For this review, take the finished solid that the model builds, in its own axes (mm). A direction names the side the tool comes from. Give positions to 0.01 mm unless a question says otherwise; leave off trailing zeros. Loops run counter-clockwise (first coordinate to the right, second up) from the corner with the lowest first, then second, coordinate; pieces in that order, holes last. Notation, with made-up numbers: (61, 27) - (108, 27) arc R26 cw to (108, 51) - close; hole circle Ø11 at (30, -19.75). An arc over 180 degrees is marked (long way). Answer as CSV lines item,"result".
from build123d import *

# Parameters (mm, degrees)
BOSS_EXTRUDE1_DEPTH = 19
BOSS_EXTRUDE2_DEPTH = 9
SKETCH2_R           = 4.5
BOSS_EXTRUDE3_DEPTH = 60
CUT_EXTRUDE1_START  = -18
CUT_EXTRUDE1_DEPTH  = 18
CUT_EXTRUDE2_START  = -68
SKETCH4_R           = 4.511504631
SKETCH4_R_2         = 4.5
CUT_EXTRUDE2_DEPTH  = 68
CUT_EXTRUDE3_DEPTH  = 34
FILLET1_R           = 10
FILLET2_R           = 3


with BuildPart() as part:
    # Sketch1 → Boss-Extrude1 (new, symmetric)
    with BuildSketch(Plane.XY):
        with BuildLine():
            Line((-36, 0), (-27, 0))
            ThreePointArc((-27, 0), (0, -27), (27, 0))
            Line((27, 0), (36, 0))
            ThreePointArc((36, 0), (0, -36), (-36, 0))
        make_face()
    extrude(amount=BOSS_EXTRUDE1_DEPTH, both=True)

    # Sketch1<3> → Boss-Extrude2 (add, symmetric)
    with BuildSketch(Plane.XY):
        with BuildLine():
            ThreePointArc((-36, 0), (0, -36), (36, 0))
            Line((36, 0), (36, -60))
            Line((36, -60), (-36, -60))
            Line((-36, -60), (-36, 0))
        make_face()
    extrude(amount=BOSS_EXTRUDE2_DEPTH, both=True)

    # Sketch2 → Boss-Extrude3 (add)
    with BuildSketch(Plane.XZ.offset(60)):
        with BuildLine():
            Line((-38, 9), (38, 9))
            ThreePointArc((38, 9), (47, 0), (38, -9))
            Line((38, -9), (-38, -9))
            ThreePointArc((-38, -9), (-47, 0), (-38, 9))
        make_face()
        with Locations((-38, 0)):
            Circle(SKETCH2_R, mode=Mode.SUBTRACT)
        with Locations((38, 0)):
            Circle(SKETCH2_R, mode=Mode.SUBTRACT)
    extrude(amount=-BOSS_EXTRUDE3_DEPTH)

    # Sketch3 → Cut-Extrude1 (cut)
    with BuildSketch(Plane(origin=(0, 0, -9), x_dir=(-1, 0, 0), z_dir=(0, 0, -1)).offset(CUT_EXTRUDE1_START)):
        with BuildLine():
            Line((27, 0), (-27, 0))
            ThreePointArc((-27, 0), (0, -27), (27, 0))
        make_face()
    extrude(amount=CUT_EXTRUDE1_DEPTH, mode=Mode.SUBTRACT)

    # Sketch4 → Cut-Extrude2 (cut)
    with BuildSketch(Plane(origin=(0, 0, 0), x_dir=(1, 0, 0), z_dir=(0, 1, 0)).offset(CUT_EXTRUDE2_START)):
        with Locations(Location((-38, 0, 0), (0, 0, 180))):
            Circle(SKETCH4_R)
        with Locations(Location((38, 0, 0), (0, 0, 90))):
            Circle(SKETCH4_R_2)
    extrude(amount=CUT_EXTRUDE2_DEPTH, mode=Mode.SUBTRACT)

    # Sketch5 → Cut-Extrude3 (cut, symmetric)
    with BuildSketch(Plane.XY):
        Polygon((-47, -60), (-22, -60), (-47, -40), align=None)
        Polygon((47, -60), (47, -40), (22, -60), align=None)
    extrude(amount=CUT_EXTRUDE3_DEPTH, both=True, mode=Mode.SUBTRACT)

    # Fillet1
    fillet1_edges = [part.edges().sort_by_distance(p)[0] for p in [
        (-22, -60, 0),
        (22, -60, 0),
    ]]
    fillet(fillet1_edges, radius=FILLET1_R)

    # Fillet2
    fillet2_edges = [part.edges().sort_by_distance(p)[0] for p in [
        (0, -36, 9),
        (0, -36, -9),
    ]]
    fillet(fillet2_edges, radius=FILLET2_R)


solid = part.part
1) Consider section A-A on z = 0. Write out the cut boundary in (x, y), and give its area (3 significant figures).
From the geometry:
outline,"(-47, -40) - (-42.51, -43.59) - (-42.51, 0) - (-47, 0) - close; (-33.49, -50.81) - (-24.74, -57.81) arc R10 ccw to (-18.49, -60) - (18.49, -60) arc R10 ccw to (24.74, -57.81) - (33.5, -50.8) - (33.5, 0) - (27, 0) arc R27 cw to (-27, 0) - (-33.49, 0) - close; (42.5, -43.6) - (47, -40) - (47, 0) - (42.5, 0) - close"
area,"3,140 mm^2"
2) Insertion check: P1, Ø4, axis at x = 13, y = -40.5, coming from the +Z side; P2, Ø3, axis at y = -7, z = -11, coming from the -X side. Each pin has a flat end and moves straight along its axis. Give the tip position at first contact, or say it passes through.
From the geometry:
P1,"stops at z = 9"
P2,"stops at x = -36.69"
3) Wall thickness on line 1 (X direction, y = -36.5, z = 0); line 2 (Z direction, x = 38, y = -15); line 3 (X direction, y = -39, z = -3): over which ranges is each line inside the solid? List them lowest first. Write a range as from..to.
From the geometry:
line 1,"x = -47..-42.51, -33.49..33.5, 42.5..47"
line 2,"z = -9..-4.5, 4.5..9"
line 3,"x = -46.49..-41.37, -34.63..34.65, 41.35..46.49"
4) Draft analysis for pull direction Z (two halves, no side actions). For faces 1 (the cylindrical face through (-33.493, -25.836, 0.198)), 2 (the cylindrical face through (47, -24, 0)), 3 (the flat face through (33.55, -50.76, 2.13)), state which applies: pulls with the +Z half, pulls with the -Z half, needs draft (parallel to the pull), parting line crosses it, or undercut.
From the geometry:
face 1,"undercut"
face 2,"parting line crosses it"
face 3,"needs draft"
5) Consider section C-C on z = -7. Write out the cut boundary in (x, y).
From the geometry:
outline,"(-43.66, -42.67) - (-24.74, -57.81) arc R10 ccw to (-18.49, -60) - (18.49, -60) arc R10 ccw to (24.74, -57.81) - (43.66, -42.67) - (43.66, 0) - (27, 0) arc R27 cw to (-27, 0) - (-43.66, 0) - close"
6) Machinability: for faces 4 (the cylindrical face through (0.79, -35.99, 15.53)), 5 (the flat face through (-32, 0, 0)), 6 (the cylindrical face through (0.79, -35.99, -15.43)), which of the approach directions +Z, -Z, +X, -X, +Y, -Y give a long, thin tool a straight path to every point of the face, cutting with its end or side? Answer none if there is none.
From the geometry:
face 4,"+Z, -Y"
face 5,"+Z, -Z, +X, -X, +Y"
face 6,"-Z, -Y"
7) Consider section D-D on z = 7.5. Write out the cut boundary in (x, y).
From the geometry:
outline,"(-42.97, -43.22) - (-24.74, -57.81) arc R10 ccw to (-18.49, -60) - (18.49, -60) arc R10 ccw to (24.74, -57.81) - (42.97, -43.22) - (42.97, 0) - (27, 0) arc R27 cw to (-27, 0) - (-42.97, 0) - close"
8) Consider section B-B on y = -18.5. Count the separate pieces of the cut face and the enclosed holes in it, and give its area (3 significant figures).
From the geometry:
separate pieces,"2"
enclosed holes,"2"
area,"1,240 mm^2"
